Geometry check sheet. Reference: the model listing, model coordinates, mm. A direction names the side the tool comes from. Coordinates: 2 decimals unless noted, no trailing zeros. Order: outer loops, then holes, each group sorted by start corner. A loop starts at its lowest first (then second) coordinate and runs counter-clockwise, first axis right, second up. Notation, with made-up numbers: (68, 29.5) - (107, 29.5) arc R25 ccw to (107, 48.5) - close; hole circle Ø2 at (36.25, 18). An arc over 180 degrees is marked (long way). One line per item, written item: value. Start each with the question number.
```python
from build123d import *

# Parameters (mm, degrees)
CROQUIS1_R              = 400
SALIENTE_EXTRUIR1_DEPTH = 520
CROQUIS3_R              = 50
CROQUIS2_R              = 400
CROQUIS4_R              = 50
SALIENTE_EXTRUIR2_DEPTH = 100
CROQUIS5_R              = 50
SALIENTE_EXTRUIR3_DEPTH = 400
CROQUIS6_W              = 100
CROQUIS6_H              = 100
SALIENTE_EXTRUIR4_DEPTH = 150


with BuildPart() as part:
    # Croquis1 → Saliente-Extruir1 (new body)
    with BuildSketch(Plane(origin=(0, 0, 0), x_dir=(1, 0, 0), z_dir=(0, 1, 0))):
        with Locations(Location((0, 0, 0), (0, 0, 270))):
            Circle(CROQUIS1_R)
    extrude(amount=-SALIENTE_EXTRUIR1_DEPTH)

    # Croquis3 → Recubrir1 section 0
    with BuildSketch(Plane(origin=(0, -900, 0), x_dir=(1, 0, 0), z_dir=(0, 1, 0))):
        Circle(CROQUIS3_R)
    # Croquis2 → Recubrir1 section 1
    with BuildSketch(Plane.XZ.offset(520)):
        Circle(CROQUIS2_R)
    loft()

    # Croquis4 → Saliente-Extruir2 (add)
    with BuildSketch(Plane.XZ.offset(900)):
        with Locations(Location((0, 0, 0), (0, 0, 270))):
            Circle(CROQUIS4_R)
    extrude(amount=SALIENTE_EXTRUIR2_DEPTH)

    # Croquis5 → Saliente-Extruir3 (add)
    with BuildSketch(Plane(origin=(0, 0, -50), x_dir=(-1, 0, 0), z_dir=(0, 0, -1))):
        with Locations((0, -950)):
            Circle(CROQUIS5_R)
    extrude(amount=-SALIENTE_EXTRUIR3_DEPTH)

    # Croquis6 → Saliente-Extruir4 (add)
    with BuildSketch(Plane(origin=(0, 0, -50), x_dir=(-1, 0, 0), z_dir=(0, 0, -1))):
        with Locations((0, -950)):
            Rectangle(CROQUIS6_W, CROQUIS6_H)
    extrude(amount=SALIENTE_EXTRUIR4_DEPTH)


solid = part.part
```
Q1. Set-up check for faces 4 (the flat face through (1, -949, 350)), 5 (the cylindrical face through (-50, -982, 0)), 6 (the flat face through (-50, -951, -124)), 7 (the flat face through (50, -951, -124)): record each of +Z, -Z, +X, -X, +Y, -Y from which the full face is reachable in a straight line by a thin tool's end or side.
Q2. Cross-section at A-A, the plane y = -281.5. Enter the section's corners in (x, z), and give its area (3 significant figures).
Q3. Gauge pin test, flat ends, axial feed: P1, Ø6, axis at y = -546, z = -128.5, coming from the +X side; P2, Ø3, axis at y = -199, z = -147, coming from the -X side; P3, Ø1.5, axis at y = -567, z = 237, coming from the +X side. Record the tip position at first contact, or that the pin passes through.
Q4. Material ranges on probe 1 along X at (y, z) = (-307.5, 13); probe 2 along X at (y, z) = (-948, 159); probe 3 along Y at (x, z) = (-13, 224.5), recorded low to high.
Q5. Release check for a two-part mould opening along Z. For faces 1 (the cylindrical face through (6.509, -900.425, 172.55)), 2 (the cylindrical face through (-50, -950, -36)), 3 (the conical face through (105.668, -834.007, -33.276)) record: released by +Z, released by -Z, zero draft, split by the parting line, or undercut.
Q6. Cross-section at B-B, the plane y = -877. Enter the section's corners in (x, z), and give its area (3 significant figures).
Check result:
1. face 4: +Z, +X, -X, -Y
1. face 5: -X, -Y
1. face 6: +Z, -Z, -X, -Y
1. face 7: +Z, -Z, +X, -Y
2. outline: circle Ø800 at (0, 0)
2. area: 503,000 mm2
3. P1: stops at x = 356.55
3. P2: stops at x = -372.6
3. P3: stops at x = 267.73
4. probe 1: x = -399.79 to 399.79
4. probe 2: x = -49.96 to 49.96
4. probe 3: y = -998.28 to -901.72, -710.13 to 0
5. face 1: zero draft
5. face 2: undercut
5. face 3: split by the parting line
6. outline: circle Ø142.37 at (0, 0)
6. area: 15,900 mm2
